from build123d import *

# Parameters (mm, degrees)
F1_DEPTH = 14
F4_DEPTH = 9
F5_DEPTH = 25.4
F6_R     = 5.08


with BuildPart() as f1:
    # F0 (on Top) → F1 (new body)
    with BuildSketch(Plane.XY):
        with BuildLine():
            Line((-22.189739, 10), (-31.439739, 10))
            ThreePointArc((-31.439739, 10), (-38.510807, 7.071068), (-41.439739, 0))
            Line((-41.439739, 0), (-30.014739, 0))
            Line((-30.014739, 0), (-30.014739, 1.443336))
            Line((-30.014739, 1.443336), (-27.364739, 4))
            Line((-27.364739, 4), (-22.189739, 4))
            Line((-22.189739, 4), (-22.189739, 10))
        make_face()
        with BuildLine():
            Line((-30.014739, 0), (-41.439739, 0))
            ThreePointArc((-41.439739, 0), (-38.510807, -7.071068), (-31.439739, -10))
            Line((-31.439739, -10), (-22.189739, -10))
            Line((-22.189739, -10), (-22.189739, -4))
            Line((-22.189739, -4), (-27.364739, -4))
            Line((-27.364739, -4), (-30.014739, -1.556664))
            Line((-30.014739, -1.556664), (-30.014739, 0))
        make_face()
        with BuildLine():
            Line((-12.939739, 10), (-22.189739, 10))
            Line((-22.189739, 10), (-22.189739, 4))
            Line((-22.189739, 4), (-14.364739, 4))
            Line((-14.364739, 4), (-14.364739, 0))
            Line((-14.364739, 0), (-2.939739, 0))
            ThreePointArc((-2.939739, 0), (-5.868671, 7.071068), (-12.939739, 10))
        make_face()
        with BuildLine():
            Line((-22.189739, -4), (-22.189739, -10))
            Line((-22.189739, -10), (-12.939739, -10))
            ThreePointArc((-12.939739, -10), (-5.868671, -7.071068), (-2.939739, 0))
            Line((-2.939739, 0), (-14.364739, 0))
            Line((-14.364739, 0), (-14.364739, -4))
            Line((-14.364739, -4), (-22.189739, -4))
        make_face()
    extrude(amount=F1_DEPTH)

    # F3 (on offset) → F4 (join)
    with BuildSketch(Plane.XY.offset(14)):
        with BuildLine():
            Line((-12.939739, 15), (-31.439739, 15))
            ThreePointArc((-31.439739, 15), (-46.439739, 0), (-31.439739, -15))
            Line((-31.439739, -15), (-12.939739, -15))
            ThreePointArc((-12.939739, -15), (2.060261, 0), (-12.939739, 15))
        make_face()
    extrude(amount=-F4_DEPTH)

    # F4_face (on face) → F5 (cut)
    with BuildSketch(Plane(origin=(-21.801895, -0.002955, 5), x_dir=(1, 0, 0), z_dir=(0, 0, -1))):
        Polygon((-8.212843, -1.446291), (-5.562843, -4.002955), (7.437157, -4.002955), (7.437157, 3.997045), (-5.562843, 3.997045), (-8.212843, 1.553709), align=None)
    extrude(amount=-F5_DEPTH, mode=Mode.SUBTRACT)

    # F6
    f6_edges = [f1.edges().sort_by_distance(p)[0] for p in [
        (-22.189739, -15, 14),
    ]]
    fillet(f6_edges, radius=F6_R)


solid = f1.part
The listing builds one solid part. Answer for the finished solid, in the listing's coordinates (mm). A direction names the side the tool comes from. Round coordinates to 2 decimals unless told otherwise and drop trailing zeros. Write each loop counter-clockwise with the first axis right and the second up, starting at its lowest first coordinate (ties: lowest second). Pieces come first, ordered by that corner, then holes. Notation, with made-up numbers: M -18.5,14 L 38.5,14 A27 ccw 38.5,30 Z; hole C 10.25,-36 d3. An arc over 180 degrees is marked long. Write each question's results on one line, items separated by ' | '. Start each with the question number.
Item 1: Which of the six approach directions +Z, -Z, +X, -X, +Y, -Y give full straight-line access (tool end or side, diameter ignored) to faces 4 (the flat face through (-28.71, 2.7, 9.44)), 5 (the flat face through (-22, -15, 7))?
Item 2: Straight lines are drawn through the part: probe 1 along Y at (x, z) = (-18, 2.25); probe 2 along Y at (x, z) = (-16.5, 8.25); probe 3 along Z at (x, y) = (-43.5, 4.5). For each, find the intervals that lie inside material, in ascending order.
Item 3: Given pin 1 Ø0.9 at (y, z) = (0.5, 2.5) entering from +X; pin 2 Ø1 at (x, z) = (-4.5, 1.5) entering from -Y; pin 3 Ø1 at (x, y) = (-33, 10.5) entering from -Z, each flat-ended and moving along its own axis, determine where each tip first touches the part or whether it passes through.
Item 4: Find section B-B on z = 6.5. Write down the section's boundary in (x, y), and give its area (3 significant figures).
Item 5: Find section A-A on x = -24.5. Write down the section's boundary in (y, z), and give its area (3 significant figures).
Item 6: Find section C-C on z = 10.25. Write down the section's boundary in (x, y).
Item 7: The mould has two halves that part along Y. Classify faces 1 (the flat face through (-22, 5, 0)), 2 (the flat face through (-28.671, -2.795, 9.437)), 3 (the flat face through (-22, -10, 2)): +Y half, -Y half, draft (parallel to the pull), parting line (faces both ways), or undercut.
Answer block:
1) face 4: +Z, -Z | face 5: +Z, -Z, +X, -X, -Y
2) probe 1: y = -10 to -4, 4 to 10 | probe 2: y = -15 to -4, 4 to 15 | probe 3: z = 5 to 13.05
3) pin 1: stops at x = -2.94 | pin 2: stops at y = -6.08 | pin 3: stops at z = 5
4) outline: M -31.44,-15 L -12.94,-15 A15 ccw -12.94,15 L -31.44,15 A15 ccw Z; hole M -30.01,-1.56 L -27.36,-4 L -14.36,-4 L -14.36,4 L -27.36,4 L -30.01,1.44 Z | area: 1,140 mm²
5) outline: M -15,5 L -10,5 L -10,0 L -4,0 L -4,14 L -9.92,14 A5.08 ccw -15,8.92 Z; M 4,0 L 10,0 L 10,5 L 15,5 L 15,8.92 A5.08 ccw 9.92,14 L 4,14 Z | area: 247 mm²
6) outline: M -31.44,-14.82 L -12.94,-14.82 A14.82 ccw -12.94,14.82 L -31.44,14.82 A14.82 ccw Z; hole M -30.01,-1.56 L -27.36,-4 L -14.36,-4 L -14.36,4 L -27.36,4 L -30.01,1.44 Z
7) face 1: draft | face 2: undercut | face 3: -Y half
